Verification items for the finished model (mm, model axes). Face numbers are marked on the shaded views. Coordinates: 2 decimals unless noted, no trailing zeros. Order: outer loops, then holes, each group sorted by start corner. A loop starts at its lowest first (then second) coordinate and runs counter-clockwise, first axis right, second up. Notation, with made-up numbers: M 18.25,4.25 L 46.25,4.25 A36 cw 46.25,41.25 Z; hole C 52.5,46 d1. An arc over 180 degrees is marked long. Return JSON: item names as keys, results as strings. Group by question number.
Q1. Thickness scan on probe 1 along Z at (x, y) = (-9, -25.5); probe 2 along Z at (x, y) = (62.5, -56.5); probe 3 along X at (y, z) = (-31, 1.75). Record the ranges inside material, lowest first.
Q2. Section check B-B, the plane y = -11. Enter the section's corners in (x, z), then the cut area to 3 significant figures.
Q3. Section check A-A, the plane x = 46. Enter the section's corners in (y, z).
Q4. Mould release check, pull along X, two halves, no side actions. Record for the marked faces 1 and 2: pulls with the +X half, pulls with the -X half, needs draft (parallel to the pull), parting line crosses it, or undercut.
Q5. Go/stop test with a flat-tipped pin: pin 1 Ø5 at (x, y) = (49.5, -43) entering from +Z. Record where the tip stops, or that it passes through.
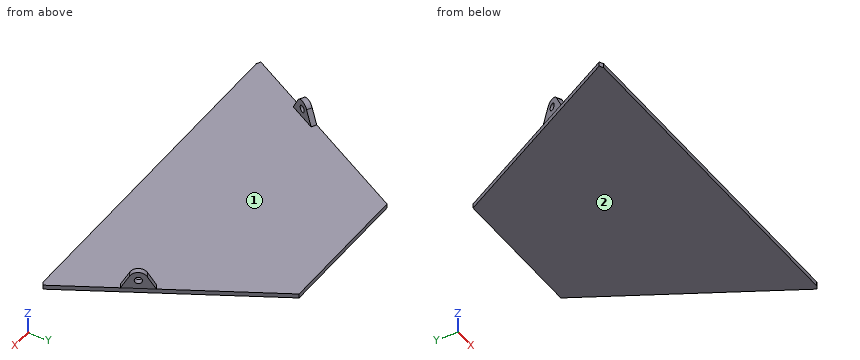
from build123d import *

# Parameters (mm, degrees)
PAD_DEPTH    = 2
SKETCH001_R  = 1.6
PAD001_DEPTH = 2.5


with BuildPart() as part:
    # Sketch → Pad (new body)
    with BuildSketch(Plane.XY):
        Polygon((-30, 0), (30, 0), (32.280434, 0), (80.027856, -87.160748), (78.273803, -88.121634), (-78.273803, -88.121634), (-80.027856, -87.160748), (-32.280434, 0), align=None)
    extrude(amount=PAD_DEPTH)

    # Sketch001 (on Face1 of Pad) → Pad001 (join)
    with BuildSketch(Plane(origin=(-24.829299, 13.601708, 0), x_dir=(-0.480443, -0.877026, 0), z_dir=(-0.877026, 0.480443, 0))):
        with BuildLine():
            Line((84.891049, 2), (70.891049, 2))
            Line((70.891049, 2), (74.444895, 8.030769))
            ThreePointArc((81.337203, 8.030769), (77.891049, 10), (74.444895, 8.030769))
            Line((84.891049, 2), (81.337203, 8.030769))
        make_face()
        with Locations((77.891049, 6)):
            Circle(SKETCH001_R, mode=Mode.SUBTRACT)
    pad001 = extrude(amount=-PAD001_DEPTH)

    # Mirrored: Pad001 across YZ
    add(pad001.mirror(Plane.YZ))


solid = part.part
Numbers:
{
 "1": {"probe 1": "z = 0 to 2", "probe 2": "z = 0 to 9.63", "probe 3": "x = -49.26 to 49.26"},
 "2": {"outline": "M -38.31,0 L 38.31,0 L 38.31,2 L -38.31,2 Z", "area": "153 mm2"},
 "3": {"outline": "M -88.12,0 L -25.04,0 L -25.04,2 L -88.12,2 Z"},
 "4": {"face 1": "undercut", "face 2": "needs draft"},
 "5": {"pin 1": "stops at z = 2"}
}
